Can you work these out from the drawing? Everything is in mm from the part's minimum corner. A direction names the side the tool comes from. Give positions to 0.01 mm unless a question says otherwise; leave off trailing zeros. Loops run counter-clockwise (first coordinate to the right, second up) from the corner with the lowest first, then second, coordinate; pieces in that order, holes last. Notation, with made-up numbers: (45.5, 56) - (50.5, 56) arc R12 cw to (50.5, 65) - close; hole circle Ø2 at (17, -28). An arc over 180 degrees is marked (long way). Write each question's results on one line, items separated by ' | '. Start each with the question number.
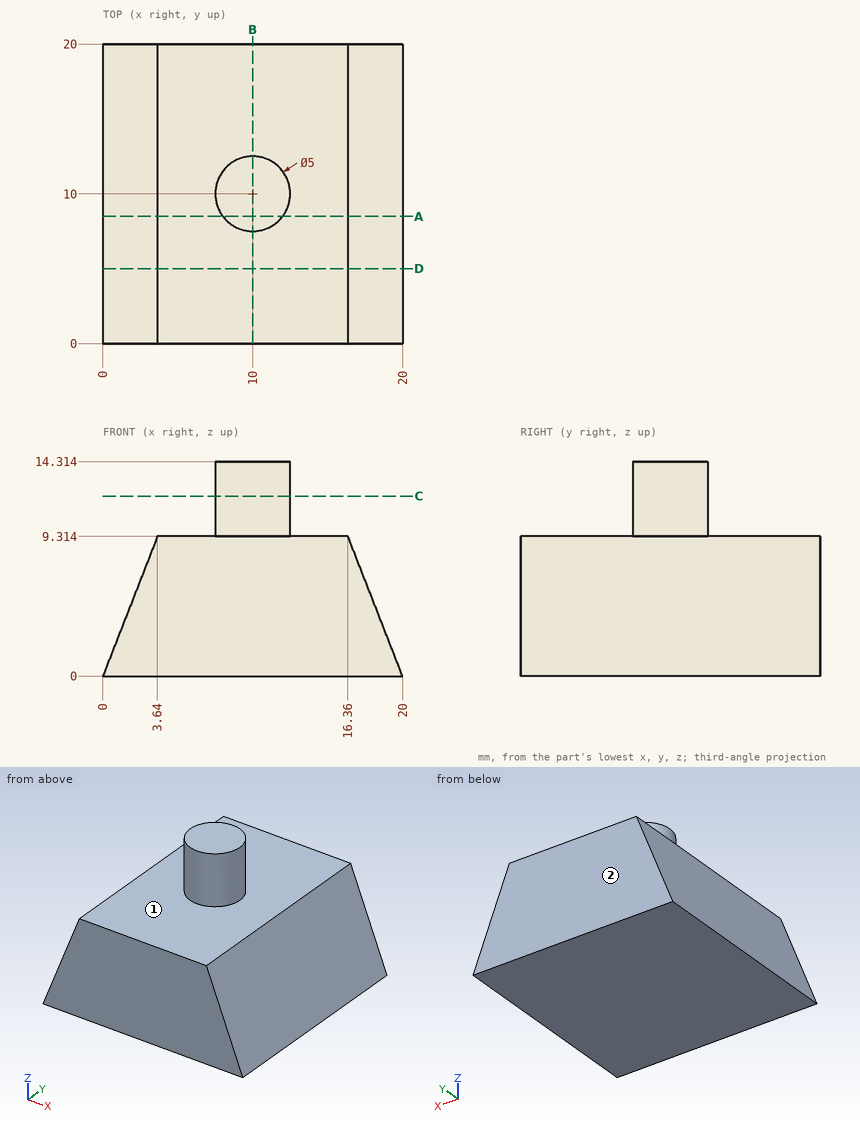
Q1. I want a section at B-B, the plane x = 10. List the corners of the cut face in (y, z) for me, then the cut area to 3 significant figures.
Q2. I want a section at D-D, the plane y = 5. List the corners of the cut face in (x, z) for me.
Q3. I want a section at A-A, the plane y = 8.5. List the corners of the cut face in (x, z) for me, then the cut area to 3 significant figures.
Q4. Which directions (+Z, -Z, +X, -X, +Y, -Y) give clear straight access to the entire face, cutting with the end or side of a thin tool? Please do the marked faces 1 and 2.
Q5. I need wall thicknesses on L1, parallel to Z at x = 14, y = 9; L2, parallel to X at y = 4.75, z = 4.5; L3, parallel to X at y = 16.5, z = 7.75. Which ranges of each line are inside material? Lowest first, please. Write a range as from..to.
Q6. I'm going to push flat-ended pins straight in: pin 1 Ø3 at (y, z) = (13, 7.5) entering from -X; pin 2 Ø3 at (y, z) = (14, 9) entering from +X; pin 3 Ø1 at (y, z) = (16.5, 11) entering from -X; pin 4 Ø2 at (x, y) = (15.5, 14) entering from +Z. Where does each tip first touch, or does it pass through?
Q7. I want a section at C-C, the plane z = 12. List the corners of the cut face in (x, y) for me, then the cut area to 3 significant figures.
Conclusion:
1) outline: (0, 0) - (20, 0) - (20, 9.31) - (12.5, 9.31) - (12.5, 14.31) - (7.5, 14.31) - (7.5, 9.31) - (0, 9.31) - close | area: 211 mm^2
2) outline: (0, 0) - (20, 0) - (16.36, 9.31) - (3.64, 9.31) - close
3) outline: (0, 0) - (20, 0) - (16.36, 9.31) - (12, 9.31) - (12, 14.31) - (8, 14.31) - (8, 9.31) - (3.64, 9.31) - close | area: 172 mm^2
4) face 1: +Z | face 2: +Z, -Z, +X, -X, +Y
5) L1: 0..9.31 | L2: 1.76..18.24 | L3: 3.03..16.97
6) pin 1: x = 2.34 | pin 2: x = 17.07 | pin 3: through | pin 4: z = 9.31
7) outline: circle Ø5 at (10, 10) | area: 19.6 mm^2
